Build history of the part. All positions in model axes, mm. Face numbers are marked on the shaded views. A direction names the side the tool comes from. Give positions to 0.01 mm unless a question says otherwise; leave off trailing zeros. Loops run counter-clockwise (first coordinate to the right, second up) from the corner with the lowest first, then second, coordinate; pieces in that order, holes last. Notation, with made-up numbers: (-22, -20.75) - (6, -20.75) arc R5 cw to (6, -16.75) - close; hole circle Ø1 at (-39.5, 5.25). An arc over 180 degrees is marked (long way). Return JSON: item names as keys, results as strings. Group by question number.
1) Slice it at C-C (z = -10). List the corners of the cut face in (x, y).
2) Slice it at A-A (x = 0). Count the separate pieces of the cut face and the enclosed holes in it, and give its area (3 significant figures).
3) Drill centre lines: probe 1 along Y at (x, z) = (3.5, 9.75); probe 2 along Y at (x, z) = (5.5, -13); probe 3 along Z at (x, y) = (0, 1.15). Where is each one in solid material? Low to high. Write a range as from..to.
4) 3-axis set-ups, long thin cutter, end or side, ignore diameter. For the marked faces 1, 2, 3, 4 and 5: which of +Z, -Z, +X, -X, +Y, -Y reach the whole face in a straight line?
5) Drop flat-ended pins along their axis: pin 1 (2.5 mm diameter, centred on x = 0, z = -10, fed in from +Y); pin 2 (2 mm diameter, centred on x = 2.5, z = -9, fed in from -Y); pin 3 (0.9 mm diameter, centred on x = 0, y = 5.5, fed in from +Z); pin 4 (5.5 mm diameter, centred on y = 7, z = 3.5, fed in from +X). Give the stop position or say it passes through.
6) Mould opens along Y. For the marked faces 6, 7 and 8 say: released by +Y, released by -Y, zero draft, split by the parting line, or undercut.
7) Slice it at B-B (y = 10.5). List the corners of the cut face in (x, z).
8) Slice it at D-D (y = 5). List the corners of the cut face in (x, z).
Autodesk Inventor part; units mm, degrees
ref_plane "YZ Plane" through (0, 0, 0) normal (1, 0, 0) x (0, 1, 0)
ref_plane "XZ Plane" through (0, 0, 0) normal (0, 1, 0) x (-1, 0, 0)
ref_plane "XY Plane" through (0, 0, 0) normal (0, 0, 1) x (1, 0, 0)
sketch "Esquisse1" plane through (0, 0, 0) normal (0, 1, 0) x (-1, 0, 0)
  line L0 (0, 0) -> (0, -15)
  line L1 (0, -15) -> (9.15, -15)
  line L2 (0, -15) -> (9.15, -15) construction
  line L3 (0, -15) -> (-9.15, -15)
  line L4 (0, 0) -> (2.55, 0)
  line L5 (0, 0) -> (-2.55, 0)
  line L6 (-2.55, 0) -> (-9.15, -15)
  line L7 (2.55, 0) -> (9.15, -15)
  line L8 (2.55, 0) -> (4.55, 0)
  line L9 (9.15, -15) -> (11.15, -15)
  line L10 (11.15, -15) -> (4.55, 0)
  line L11 (-9.15, -15) -> (-11.15, -15)
  line L12 (-2.55, 0) -> (-4.55, 0)
  line L13 (-4.55, 0) -> (-11.15, -15)
  line L14 (0, 0) -> (0, 2)
  line L15 (0, 2) -> (4.55, 2)
  line L16 (4.55, 2) -> (4.55, 0)
  line L17 (0, 2) -> (-4.55, 2)
  line L18 (-4.55, 2) -> (-4.55, 0)
  dimension "d0" = 15
  dimension "d1" = 9.15
  dimension "d2" = 0
  dimension "d3" = 9.15
  dimension "d4" = 2.55
  dimension "d5" = 2.55
  dimension "d7" = 2
  dimension "d8" = 2
  dimension "d9" = 2
  dimension "d10" = 2
  dimension "d11" = 2
extrude "Extrusion1" add sketch "Esquisse1" along normal blind 12 contours L14 L15 L16 L8 L4 | L5 L12 L18 L17 L14 | L8 L10 L9 L7 | L6 L11 L13 L12
sketch "Esquisse2" plane through (0, 0, 0) normal (0, -1, 0) x (1, 0, 0)
  line L0 (-2.55, 0) -> (-9.15, -15)
  line L1 (-2.55, 0) -> (-9.15, -15)
  line L2 (9.15, -15) -> (2.55, 0)
  line L3 (-9.15, -15) -> (9.15, -15)
  line L4 (9.15, -15) -> (2.55, 0)
  line L5 (2.55, 0) -> (-2.55, 0)
  point P0 (0, 0)
extrude "Extrusion2" add sketch "Esquisse2" against normal blind 0.99
sketch "Esquisse3" plane through (0, 12, 0) normal (0, 1, 0) x (1, 0, 0)
  line L0 (2.55, 0) -> (-2.55, 0)
  line L1 (2.55, 0) -> (-2.55, 0)
  line L2 (-9.15, 15) -> (-11.15, 15)
  line L3 (-2.55, 0) -> (-9.15, 15)
  line L4 (9.15, 15) -> (2.55, 0)
  line L5 (-9.15, 15) -> (9.15, 15)
  line L6 (9.15, 15) -> (2.55, 0)
  point P0 (0, 0)
extrude "Extrusion3" add sketch "Esquisse3" against normal blind 0.99
sketch "Esquisse4" plane through (0, 12, 0) normal (0, 1, 0) x (1, 0, 0)
  line L0 (0, 0) -> (0, 15)
  line L1 (11.15, 15) -> (-11.15, 15)
  line L2 (0, 0) -> (0, 10)
  line L3 (0, 10) -> (0, 20)
  dimension "d18" = 10
  dimension "d19" = 10
hole "Perçage1" at (0, 12, -10) at (0, 12, -20) direction (0, -1, 0) diameter 4.134 end through all
sketch "Esquisse5" plane through (0, 12, 0) normal (0, 1, 0) x (1, 0, 0)
  line L0 (-4.55, -2) -> (4.55, -2)
  line L1 (-4.55, -2) -> (-4.55, -7)
  line L2 (-4.55, -7) -> (4.55, -7)
  line L3 (4.55, -7) -> (4.55, -2)
  arc A0 (-4.55, -7) -> (4.55, -7) centre (0, -7) ccw
  point P0 (0, 0)
  dimension "d27" = 5
extrude "Extrusion4" add sketch "Esquisse5" against normal blind 2
fillet "Congé1" radius 2.5 1 edges at (0, 10, 2)
sketch "Esquisse7" plane through (0, 12, 0) normal (0, 1, 0) x (1, 0, 0)
  line L0 (4.55, -4.5) -> (-4.55, -4.5)
  line L1 (0, -4.5) -> (0, -7.0145)
  point P0 (0, 0)
  dimension "d43" = 2.5145
sketch "Esquisse8" plane through (0, 0, 0) normal (0, -1, 0) x (1, 0, 0)
  line L0 (-4.55, 2) -> (4.55, 2)
  line L1 (-4.55, 7) -> (-4.55, 2)
  line L2 (4.55, 7) -> (4.55, 0)
  line L3 (4.55, 2) -> (4.55, 7)
  line L4 (-4.55, 2) -> (4.55, 2)
  arc A0 (4.55, 7) -> (-4.55, 7) centre (0, 0.4199) ccw
  arc A1 (4.55, 7) -> (-4.55, 7) centre (0, 7) ccw
  line L5 (-4.55, 0) -> (-4.55, 7)
  point P0 (0, 0)
extrude "Extrusion5" add sketch "Esquisse8" against normal blind 2
fillet "Congé2" radius 2.5 1 edges at (0, 2, 2)
hole "Perçage2" at (0, 12, 7.0145) direction (0, -1, 0) diameter 4.134 end through all
properties part number "Fixation_rotule_axe_centrale"
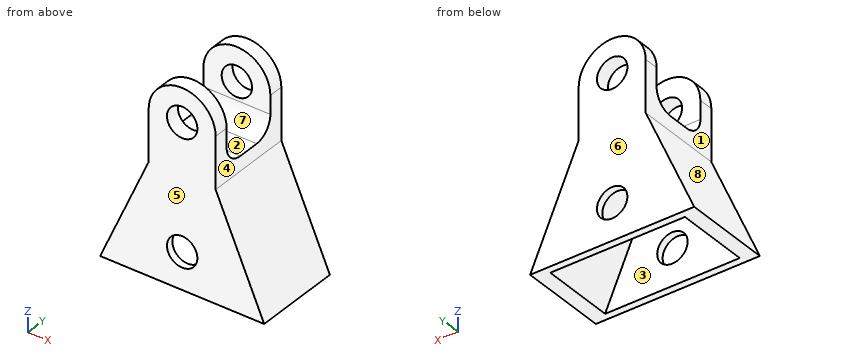
Results:
{
 "1": {"outline": "(-8.95, 0) - (-2.07, 0) - (-2.07, 0.99) - (-6.95, 0.99) - (-6.95, 11.01) - (-2.07, 11.01) - (-2.07, 12) - (-8.95, 12) - close; (2.07, 0) - (8.95, 0) - (8.95, 12) - (2.07, 12) - (2.07, 11.01) - (6.95, 11.01) - (6.95, 0.99) - (2.07, 0.99) - close"},
 "2": {"separate pieces": "5", "enclosed holes": "0", "area": "69.9 mm2"},
 "3": {"probe 1": "0..2, 10..12", "probe 2": "0..0.99, 11.01..12", "probe 3": "0..4.95, 9.08..11.55"},
 "4": {"face 1": "+Z, -X, +Y, -Y", "face 2": "+Z, +X, -X", "face 3": "-Z", "face 4": "+Z, +X, +Y, -Y", "face 5": "+Z, -Z, +X, -X, -Y"},
 "5": {"pin 1": "through", "pin 2": "y = 0", "pin 3": "z = 2", "pin 4": "x = 4.55"},
 "6": {"face 6": "released by +Y", "face 7": "undercut", "face 8": "zero draft"},
 "7": {"outline": "(-11.15, -15) - (-9.15, -15) - (-2.55, 0) - (2.55, 0) - (9.15, -15) - (11.15, -15) - (4.55, 0) - (4.55, 7) arc R4.55 ccw to (-4.55, 7) - (-4.55, 0) - close; hole circle Ø4.13 at (0, 7.01)"},
 "8": {"outline": "(-11.15, -15) - (-9.15, -15) - (-2.55, 0) - (2.55, 0) - (9.15, -15) - (11.15, -15) - (4.55, 0) - (4.55, 2) - (-4.55, 2) - (-4.55, 0) - close"}
}
